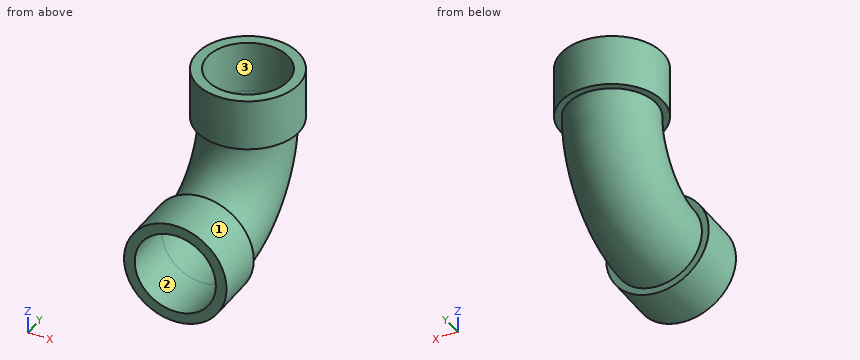
from build123d import *

# Parameters (mm, degrees)
SKETCH1_R           = 38.1
SKETCH1_R_2         = 30.1625
BOSS_EXTRUDE1_DEPTH = 38.1
SKETCH4_R           = 38.1
SKETCH4_R_2         = 30.1625
BOSS_EXTRUDE2_DEPTH = 38.1
SKETCH6_R           = 33.02
SKETCH6_R_2         = 30.1625


with BuildPart() as part:
    # Sketch1 → Boss-Extrude1 (new body)
    with BuildSketch(Plane(origin=(0, 0, 0), x_dir=(1, 0, 0), z_dir=(0, 1, 0))):
        Circle(SKETCH1_R)
        Circle(SKETCH1_R_2, mode=Mode.SUBTRACT)
    extrude(amount=BOSS_EXTRUDE1_DEPTH)



with BuildPart() as body_2:
    # Sketch4 → Boss-Extrude2 (new body)
    with BuildSketch(Plane.XY.offset(63.5)):
        with Locations((0, 101.6)):
            Circle(SKETCH4_R)
        with Locations((0, 101.6)):
            Circle(SKETCH4_R_2, mode=Mode.SUBTRACT)
    extrude(amount=BOSS_EXTRUDE2_DEPTH)


with BuildPart() as part_1:
    add(part.part)

    add(body_2.part)  # Sweep2 merges body 2
    # Sweep2: sweep along a path in Sketch3
    with BuildLine(Plane(origin=(0, 0, 0), x_dir=(0, 0, -1), z_dir=(1, 0, 0))) as sweep2_path:
        ThreePointArc((0, 38.1), (-18.598719395, 83.001280605), (-63.5, 101.6))
    # Sketch6 → Sweep2 (sweep)
    with BuildSketch(Plane(origin=(0, 38.1, 0), x_dir=(1, 0, 0), z_dir=(0, 1, 0))):
        Circle(SKETCH6_R)
        Circle(SKETCH6_R_2, mode=Mode.SUBTRACT)
    sweep(path=sweep2_path.line)


solid = part_1.part
Source: CAD feature listing. Evaluate the final solid. Frame: model axes, mm. Face numbers are marked on the shaded views. Give positions to 0.01 mm unless a question says otherwise; leave off trailing zeros. Order: outer loops, then holes, each group sorted by start corner. A loop starts at its lowest first (then second) coordinate and runs counter-clockwise, first axis right, second up. Notation, with made-up numbers: (36.25, -31) -> (42.25, -31) arc R18 ccw to (42.25, -18) -> close; hole circle Ø1 at (48.25, 57). An arc over 180 degrees is marked (long way). Write item = value, one per line.
Q1. Material intervals for line 1 (X direction, y = 101, z = 83); line 2 (Y direction, x = 0, z = 83), sorted ascending. Write a range as from..to.
Data:
line_1 = -38.1..-30.16, 30.16..38.1
line_2 = 63.5..71.44, 131.76..139.7
Q2. Pin query (flat end, axial travel): pin 1 (3 mm diameter, centred on x = -13.5, z = 64.5, fed in from -Y); pin 2 (5 mm diameter, centred on x = -1, z = 48, fed in from +Y); pin 3 (8 mm diameter, centred on x = -22.5, y = 21.5, fed in from -Z). Return the tip coordinate at first contact, or that it passes through.
Data:
pin_1 = 65.44
pin_2 = 133.73
pin_3 = -33.31
Q3. Cut plane B-B, the plane x = -26.5. Output: boundary loops of the cut face in (y, z), and give its area (3 significant figures).
Data:
outline = (0, -27.37) -> (38.1, -27.37) -> (38.1, -19.7) arc R83.2 ccw to (121.3, 63.5) -> (128.97, 63.5) -> (128.97, 101.6) -> (116.01, 101.6) -> (116.01, 63.5) arc R77.91 cw to (38.1, -14.41) -> (0, -14.41) -> close; (0, 14.41) -> (38.1, 14.41) arc R49.09 ccw to (87.19, 63.5) -> (87.19, 101.6) -> (74.23, 101.6) -> (74.23, 63.5) -> (81.9, 63.5) arc R43.8 cw to (38.1, 19.7) -> (38.1, 27.37) -> (0, 27.37) -> close
area = 3,030 mm^2
Q4. Pull-direction query (Z, two-part tool) for the marked faces 1, 2 and 3; classes: released by +Z, released by -Z, zero draft, split by the parting line, or undercut.
Data:
face_1 = split by the parting line
face_2 = undercut
face_3 = zero draft
Q5. Cut plane A-A, the plane x = 0. Output: boundary loops of the cut face in (y, z) (1 decimal), and give its area (3 significant figures).
Data:
outline = (0, -38.1) -> (38.1, -38.1) -> (38.1, -33) arc R96.5 ccw to (134.6, 63.5) -> (139.7, 63.5) -> (139.7, 101.6) -> (131.8, 101.6) -> (131.8, 63.5) arc R93.7 cw to (38.1, -30.2) -> (0, -30.2) -> close; (0, 30.2) -> (38.1, 30.2) arc R33.3 ccw to (71.4, 63.5) -> (71.4, 101.6) -> (63.5, 101.6) -> (63.5, 63.5) -> (68.6, 63.5) arc R30.5 cw to (38.1, 33) -> (38.1, 38.1) -> (0, 38.1) -> close
area = 1,780 mm^2
